Build history of the part. All positions in model axes, mm. Face numbers are marked on the shaded views. A direction names the side the tool comes from. Round coordinates to 2 decimals unless told otherwise and drop trailing zeros. Order: outer loops, then holes, each group sorted by start corner. A loop starts at its lowest first (then second) coordinate and runs counter-clockwise, first axis right, second up. Notation, with made-up numbers: (-21.75, 28.5) -> (9.25, 28.5) arc R22 cw to (9.25, 53.5) -> close; hole circle Ø8 at (43, 64.25). An arc over 180 degrees is marked (long way). Use a Markdown table: item, result. Add a question column.
Item 1: Probe L1, parallel to X at y = 42, z = -5; L2, parallel to Z at x = 2, y = 65. List the from-to ranges inside material, lowest first.
Item 2: 3-axis set-ups, long thin cutter, end or side, ignore diameter. For the marked faces 5, 6 and 7: which of +Z, -Z, +X, -X, +Y, -Y reach the whole face in a straight line?
Item 3: Slice it at D-D, the plane z = -17. Give the cut face in (x, y), plus the area to 3 significant figures.
Item 4: Slice it at C-C, the plane y = 82. Give the cut face in (x, z), plus the area to 3 significant figures.
Item 5: Slice it at A-A, the plane x = 0. State how many separate pieces and enclosed holes the cut face has, plus the area to 3 significant figures.
Item 6: Pin check, flat tips, straight feed: pin 1 (4.5 mm diameter, centred on x = 0, y = 19.64, fed in from -Z); pin 2 (4 mm diameter, centred on x = -1.5, z = 7.5, fed in from -Y); pin 3 (16.5 mm diameter, centred on x = -4, y = 21, fed in from +Z). Stop position of each tip, or through.
Item 7: Two-plate mould, pull along Z, no slides. Class the marked faces 1, 2, 3 and 4: released by +Z, released by -Z, zero draft, split by the parting line, or undercut.
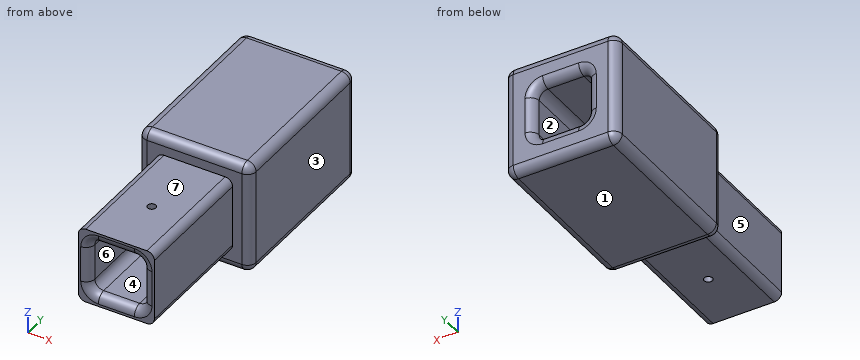
from build123d import *

# Parameters (mm, degrees)
SKETCH1_W           = 25.781
SKETCH1_H           = 25.781
SKETCH1_W_2         = 18.161
SKETCH1_H_2         = 18.161
BOSS_EXTRUDE1_DEPTH = 101.6
BOSS_EXTRUDE2_START = 43.4
SKETCH1_3_W         = 38.1
SKETCH1_3_H         = 38.1
SKETCH1_3_W_2       = 25.781
SKETCH1_3_H_2       = 25.781
BOSS_EXTRUDE2_DEPTH = 58.2
FILLET1_R           = 2.54
FILLET2_R           = 2.9845
SKETCH2_R           = 1.4
CUT_EXTRUDE1_DEPTH  = 37.592


with BuildPart() as part:
    # Sketch1 → Boss-Extrude1 (new body)
    with BuildSketch(Plane(origin=(0, 0, 0), x_dir=(1, 0, 0), z_dir=(0, 1, 0))):
        Rectangle(SKETCH1_W, SKETCH1_H)
        Rectangle(SKETCH1_W_2, SKETCH1_H_2, mode=Mode.SUBTRACT)
    extrude(amount=BOSS_EXTRUDE1_DEPTH)

    # Sketch1<3> → Boss-Extrude2 (add)
    with BuildSketch(Plane(origin=(0, 0, 0), x_dir=(1, 0, 0), z_dir=(0, 1, 0)).offset(BOSS_EXTRUDE2_START)):
        Rectangle(SKETCH1_3_W, SKETCH1_3_H)
        Rectangle(SKETCH1_3_W_2, SKETCH1_3_H_2, mode=Mode.SUBTRACT)
    extrude(amount=BOSS_EXTRUDE2_DEPTH)

    # Fillet1
    fillet1_edges = [part.edges().sort_by_distance(p)[0] for p in [
        (-12.8905, 21.7, -12.8905),
        (12.8905, 21.7, -12.8905),
        (12.8905, 21.7, 12.8905),
        (-12.8905, 21.7, 12.8905),
    ]]
    fillet(fillet1_edges, radius=FILLET1_R)

    # Fillet2
    fillet2_edges = [part.edges().sort_by_distance(p)[0] for p in [
        (0, 0, 9.0805),
        (9.0805, 0, 0),
        (9.0805, 50.8, -9.0805),
        (-9.0805, 50.8, -9.0805),
        (-9.0805, 50.8, 9.0805),
        (9.0805, 50.8, 9.0805),
        (9.0805, 101.6, 0),
        (0, 101.6, 9.0805),
        (19.05, 72.5, -19.05),
        (0, 43.4, -19.05),
        (19.05, 72.5, 19.05),
        (19.05, 43.4, 0),
        (0, 101.6, 19.05),
        (-19.05, 72.5, 19.05),
        (-19.05, 101.6, 0),
        (-19.05, 72.5, -19.05),
        (-9.0805, 101.6, 0),
        (-19.05, 43.4, 0),
        (0, 43.4, 19.05),
        (19.05, 101.6, 0),
        (0, 101.6, -19.05),
        (0, 101.6, -9.0805),
        (0, 0, -9.0805),
        (-9.0805, 0, 0),
    ]]
    fillet(fillet2_edges, radius=FILLET2_R)

    # Sketch2 → Cut-Extrude1 (cut)
    with BuildSketch(Plane(origin=(0, 0, -12.8905), x_dir=(-1, 0, 0), z_dir=(0, 0, -1))):
        with Locations((0, 19.643054378)):
            Circle(SKETCH2_R)
    extrude(amount=-CUT_EXTRUDE1_DEPTH, mode=Mode.SUBTRACT)


solid = part.part
Check sheet entries:
| question | item | result |
|---|---|---|
| 1 | L1 | -12.89 to -9.08, 9.08 to 12.89 |
| 1 | L2 | -19.05 to -9.08, 9.08 to 19.05 |
| 2 | face 5 | +Z, -Z, -X, -Y |
| 2 | face 6 | +Y, -Y |
| 2 | face 7 | +Z, +X, -X, -Y |
| 3 | outline | (-18.9, 46.38) arc R2.83 ccw to (-16.07, 43.55) -> (16.07, 43.55) arc R2.83 ccw to (18.9, 46.38) -> (18.9, 98.62) arc R2.83 ccw to (16.07, 101.45) -> (-16.07, 101.45) arc R2.83 ccw to (-18.9, 98.62) -> close |
| 3 | area | 2,180 mm2 |
| 4 | outline | (-19.05, -16.07) arc R2.98 ccw to (-16.07, -19.05) -> (16.07, -19.05) arc R2.98 ccw to (19.05, -16.07) -> (19.05, 16.07) arc R2.98 ccw to (16.07, 19.05) -> (-16.07, 19.05) arc R2.98 ccw to (-19.05, 16.07) -> close; hole (-9.08, -6.1) arc R2.98 ccw to (-6.1, -9.08) -> (6.1, -9.08) arc R2.98 ccw to (9.08, -6.1) -> (9.08, 6.1) arc R2.98 ccw to (6.1, 9.08) -> (-6.1, 9.08) arc R2.98 ccw to (-9.08, 6.1) -> close |
| 4 | area | 1,120 mm2 |
| 5 | separate pieces | 4 |
| 5 | enclosed holes | 0 |
| 5 | area | 1,450 mm2 |
| 6 | pin 1 | z = -12.89 |
| 6 | pin 2 | y = 1.46 |
| 6 | pin 3 | z = 12.89 |
| 7 | face 1 | released by -Z |
| 7 | face 2 | undercut |
| 7 | face 3 | zero draft |
| 7 | face 4 | undercut |
